Geometry check sheet. Reference: the model listing, model coordinates, mm. A direction names the side the tool comes from. Coordinates: 2 decimals unless noted, no trailing zeros. Write each loop counter-clockwise with the first axis right and the second up, starting at its lowest first coordinate (ties: lowest second). Pieces come first, ordered by that corner, then holes. Notation, with made-up numbers: (-6, 74.5) -> (36, 74.5) arc R28 ccw to (36, 113.5) -> close; hole circle Ø4 at (5, 5.25). An arc over 180 degrees is marked (long way). One line per question, with ' | ' between items.
```python
from build123d import *

# Parameters (mm, degrees)
F1_DEPTH = 2.5
F2_W     = 0.4
F2_H     = 3.67
F3_DEPTH = 4.5
F4_W     = 3.4
F4_H     = 1
F5_DEPTH = 25
F6_R     = 1.33499


# Not quite as in the source:
# - a fillet or chamfer is up to 0.001 mm smaller than in the source, because OpenCascade refuses the exact size
# - ends of sketch curves that miss each other by under 0.0002 mm in the source are joined


with BuildPart() as f1:
    # F0 (on Front) → F1 (new body)
    with BuildSketch(Plane.XZ):
        with BuildLine():
            Line((0.71, 1.835), (0.71, -1.835))
            Line((0.71, -1.835), (1.11, -1.835))
            Line((1.11, -1.835), (1.11, 1.835))
            ThreePointArc((1.11, 1.835), (0, 2.945), (-1.11, 1.835))
            Line((-1.11, 1.835), (-1.11, -2.3328240747))
            ThreePointArc((-1.11, -2.3328240747), (-1.421083088, -2.8586837383), (-2.031758919, -2.8392524256))
            Line((-2.031758919, -2.8392524256), (-6.6740188024, 0.1102260326))
            Line((-6.6740188024, 0.1102260326), (-6.8885263266, -0.227392868))
            Line((-6.8885263266, -0.227392868), (-2.2462664432, -3.1768713262))
            ThreePointArc((-2.2462664432, -3.1768713262), (-1.2294272033, -3.2097802095), (-0.71, -2.335))
            Line((-0.71, -2.335), (-0.71, 1.835))
            ThreePointArc((-0.71, 1.835), (0, 2.545), (0.71, 1.835))
        make_face()
    extrude(amount=F1_DEPTH)

    # F2 (on face) → F3 (join)
    with BuildSketch(Plane.XZ.offset(2.5)):
        with Locations((0.91, 0)):
            Rectangle(F2_W, F2_H)
    extrude(amount=F3_DEPTH)

    # F4 (on face) → F5 (cut)
    with BuildSketch(Plane.YZ.offset(1.11)):
        with Locations((-5.3, -1.335)):
            Rectangle(F4_W, F4_H)
    extrude(amount=-F5_DEPTH, mode=Mode.SUBTRACT)

    # F6 (radius 1.335 in the source; OpenCascade refuses exactly that, so slightly less here)
    f6_edges = [f1.edges().sort_by_distance(p)[0] for p in [
        (0.91, -7, 1.835),
        (0.91, -7, -0.835),
    ]]
    fillet(f6_edges, radius=F6_R)


solid = f1.part
```
(1) Depth check by flat-ended pin: P1, Ø1.8, axis at y = -4.5, z = -0.5, coming from the -X side; P2, Ø3, axis at y = -1.5, z = -1, coming from the -X side; P3, Ø3, axis at x = -1, z = -1.5, coming from the -Y side; P4, Ø3, axis at y = -5, z = -2.5, coming from the -X side. Enter the tip coordinate at first touch or a pass-through.
Answers below:
P1: stops at x = 0.71 | P2: stops at x = -6.89 | P3: stops at y = -2.5 | P4: passes through
(2) Cross-section at C-C (z = -0.5). Record the cut outline in (x, y), plus the area to 3 significant figures.
Answers below:
outline: (-6.46, -2.5) -> (-5.71, -2.5) -> (-5.71, 0) -> (-6.46, 0) -> close; (-1.11, -2.5) -> (-0.71, -2.5) -> (-0.71, 0) -> (-1.11, 0) -> close; (0.71, -6.55) -> (1.11, -6.55) -> (1.11, 0) -> (0.71, 0) -> close | area: 5.48 mm²
(3) Cross-section at A-A (z = 2.25). Record the cut outline in (x, y).
Answers below:
outline: (-1.03, -2.5) -> (-0.58, -2.5) -> (-0.58, 0) -> (-1.03, 0) -> close; (0.58, -2.5) -> (1.03, -2.5) -> (1.03, 0) -> (0.58, 0) -> close
(4) Material ranges on line 1 (X direction, y = -0.75, z = 0); line 2 (X direction, y = -3, z = -1.25); line 3 (X direction, y = -2, z = 2.25), recorded low to high.
Answers below:
line 1: x = -6.74 to -6.5, -1.11 to -0.71, 0.71 to 1.11 | line 2: x = 0.71 to 1.11 | line 3: x = -1.03 to -0.58, 0.58 to 1.03
(5) Cross-section at D-D (x = 0). Record the cut outline in (y, z) (3 decimals).
Answers below:
outline: (-2.5, 2.545) -> (0, 2.545) -> (0, 2.945) -> (-2.5, 2.945) -> close
(6) Tool access check on faces 5 (the face through (1.11, -3, 0)), 6 (the face through (-1.11, -1, 0)), 7 (the face through (-0.71, -1, 0)). Record the directions out of +Z, -Z, +X, -X, +Y, -Y that give a thin tool (end or side, any length) a straight path to the whole face; none if there is none.
Answers below:
face 5: +Z, -Z, +X, +Y, -Y | face 6: +Z, +Y, -Y | face 7: -Z, +Y, -Y
(7) Draft check along X on faces 1 (the face through (0.913, -6.599, 1.454)), 2 (the face through (-4.6, -1.23, -1.68)), 3 (the face through (-4.3, -1.2, -1.4)), 4 (the face through (-1.413, -1.232, -2.854)). Enter one of: pulls with the +X half, pulls with the -X half, needs draft (parallel to the pull), parting line crosses it, or undercut.
Answers below:
face 1: needs draft | face 2: pulls with the -X half | face 3: undercut | face 4: undercut
(8) Cross-section at B-B (y = -1.5). Record the cut outline in (x, z) (3 decimals).
Answers below:
outline: (-6.889, -0.227) -> (-2.246, -3.177) arc R1 ccw to (-0.71, -2.335) -> (-0.71, 1.835) arc R0.71 cw to (0.71, 1.835) -> (0.71, -1.835) -> (1.11, -1.835) -> (1.11, 1.835) arc R1.11 ccw to (-1.11, 1.835) -> (-1.11, -2.333) arc R0.6 cw to (-2.032, -2.839) -> (-6.674, 0.11) -> close
